The model under review builds one solid part; all positions refer to its coordinate system, in mm. Face numbers are marked on the shaded views. A direction names the side the tool comes from. Coordinates: 2 decimals unless noted, no trailing zeros. Loops run counter-clockwise (first coordinate to the right, second up) from the corner with the lowest first, then second, coordinate; pieces in that order, holes last. Notation, with made-up numbers: M 32,33 L 55,33 A32 ccw 55,70 Z; hole C -10,-13 d7. An arc over 180 degrees is marked long. Write item = value, one per line. Start each with the question number.
Q1. Wall thickness on probe 1 along X at (y, z) = (81.5, 15); probe 2 along Z at (x, y) = (-1, -50.5); probe 3 along Y at (x, z) = (-39.5, 20.75): over which ranges is each line inside the solid? List them lowest first.
Q2. Clearance check with flat-ended pins moving along their axes: pin 1 Ø6 at (y, z) = (-10.5, 15) entering from +X; pin 2 Ø12.5 at (y, z) = (85.5, 8.5) entering from -X; pin 3 Ø12.5 at (x, y) = (-55, -54.5) entering from +Z; pin 4 Ø12 at (x, y) = (-45.5, 26.5) entering from +Z. State where each tip first meets the part, or that it passes through.
Q3. We need section D-D on y = 28. Give the boundary of the cut face in (x, z).
Q4. We need section A-A on y = 69. Give the boundary of the cut face in (x, z).
Q5. Mouldability with a two-part tool opening along X and no side actions: class the marked faces 6, 7 and 8 as released by +X, released by -X, zero draft, split by the parting line, or undercut.
Q6. We need section B-B on z = 10.25. Give the boundary of the cut face in (x, y).
Q7. For the marked faces 1, 2, 3, 4 and 5, list the 3-axis set-ups (+Z, -Z, +X, -X, +Y, -Y) from which the entire face can be reached by the end or side of a thin tool; tool diameter is ignored.
Q8. We need section C-C on x = 19. Give the boundary of the cut face in (y, z).
from build123d import *

# Parameters (mm, degrees)
F0_W     = 69.0733827651
F0_H     = 95.5515131354
F1_DEPTH = 25.4
F2_W     = 28.6007858813
F2_H     = 25.4682730883
F2_W_2   = 28.9632454515
F2_H_2   = 25.2022650093
F3_DEPTH = 25.4
F4_W     = 53.2440617681
F4_H     = 25.4
F5_DEPTH = 9.144
F6_W     = 53.2063767314
F6_H     = 25.4
F7_DEPTH = 6.604


with BuildPart() as f1:
    # F0 (on Top) → F1 (new body)
    with BuildSketch(Plane.XY):
        with Locations((0.1439023763, -0.1439042389)):
            Rectangle(F0_W, F0_H)
    extrude(amount=F1_DEPTH)

    # F2 (on face) → F3 (join)
    with BuildSketch(Plane.XZ.offset(47.9196608067)):
        with Locations((48.9809866995, 12.7341365442)):
            Rectangle(F2_W, F2_H)
        with Locations((-48.874411732, 12.6011325046)):
            Rectangle(F2_W_2, F2_H_2)
        Polygon((-34.3927890062, 0), (34.6805937588, 0), (34.6805937588, 25.4), (-34.3927890062, 25.4), (-34.3927890062, 25.2022650093), align=None)
    extrude(amount=F3_DEPTH)

    # F4 (on face) → F5 (join)
    with BuildSketch(Plane.YZ.offset(34.6805937588)):
        with Locations((74.2538832128, 12.7)):
            Rectangle(F4_W, F4_H)
    extrude(amount=-F5_DEPTH)

    # F6 (on face) → F7 (join)
    with BuildSketch(Plane(origin=(-34.3927890062, 0, 0), x_dir=(0, -1, 0), z_dir=(-1, 0, 0))):
        with Locations((-74.2350406945, 12.7)):
            Rectangle(F6_W, F6_H)
    extrude(amount=-F7_DEPTH)


solid = f1.part
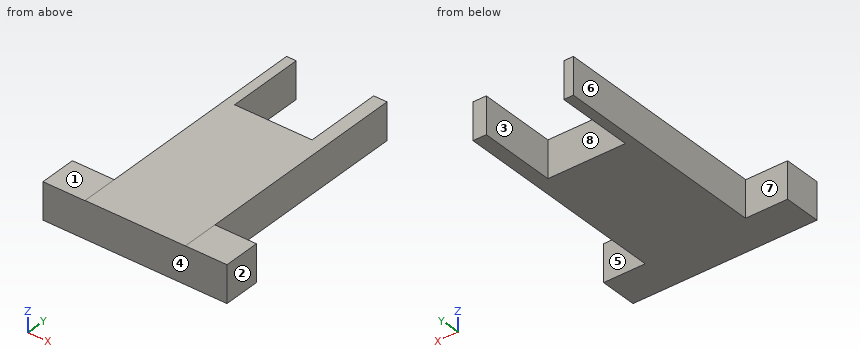
Returned:
q1.probe_1 = -34.39 to -27.79, 25.54 to 34.68
q1.probe_2 = 0 to 25.4
q1.probe_3 = -73.32 to -47.92
q2.pin_1 = 34.68
q2.pin_2 = -34.39
q2.pin_3 = 25.2
q2.pin_4 = through
q3.outline = M -34.39,0 L 34.68,0 L 34.68,25.4 L -34.39,25.4 Z
q4.outline = M -34.39,0 L -27.79,0 L -27.79,25.4 L -34.39,25.4 Z; M 25.54,0 L 34.68,0 L 34.68,25.4 L 25.54,25.4 Z
q5.face_6 = released by -X
q5.face_7 = zero draft
q5.face_8 = undercut
q6.outline = M -63.36,-73.32 L 63.28,-73.32 L 63.28,-47.92 L 34.68,-47.92 L 34.68,100.88 L 25.54,100.88 L 25.54,47.63 L -27.79,47.63 L -27.79,100.84 L -34.39,100.84 L -34.39,-47.92 L -63.36,-47.92 Z
q7.face_1 = +Z, -X, +Y, -Y
q7.face_2 = +Z, -Z, +X, +Y, -Y
q7.face_3 = +Z, -Z, +Y
q7.face_4 = +Z, -Z, +X, -X, -Y
q7.face_5 = +Z, -Z, +X, +Y
q8.outline = M -73.32,0 L 47.63,0 L 47.63,25.4 L -73.32,25.4 Z
